Build history of the part. All positions in model axes, mm. Give positions to 0.01 mm unless a question says otherwise; leave off trailing zeros. Write each loop counter-clockwise with the first axis right and the second up, starting at its lowest first coordinate (ties: lowest second). Pieces come first, ordered by that corner, then holes.
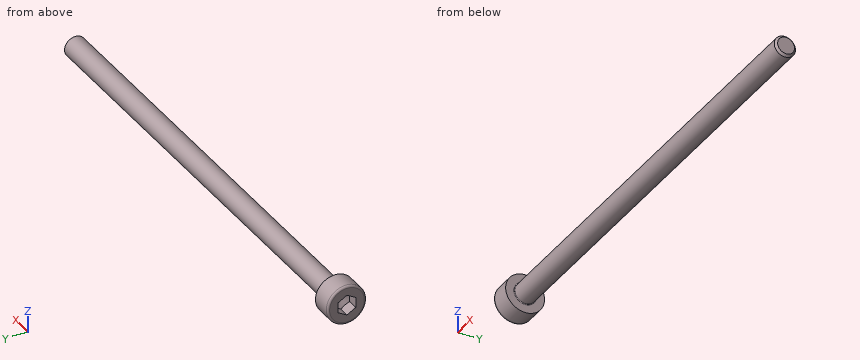
Autodesk Inventor part; units mm, degrees
ref_plane "Work Plane1" through (29, 0, 0) normal (0, -1, 0) x (1, 0, 0)
ref_plane "YZ Plane" through (0, 0, 0) normal (1, 0, 0) x (0, 1, 0)
ref_plane "XZ Plane" through (0, 0, 0) normal (0, 1, 0) x (-1, 0, 0)
sketch "Sketch1" plane through (0, 0, 0) normal (0, 0, 1) x (1, 0, 0)
  line L0 (-0.6667, 0) -> (65, 0)
  line L1 (65, 0) -> (65, 1.5)
  line L2 (65, 1.5) -> (47, 1.5)
  line L3 (47, 1.5) -> (46.6932, 1.5)
  line L4 (46.6932, 1.5) -> (0, 1.5)
  line L5 (0, 1.5) -> (0, 2.75)
  line L6 (0, 2.75) -> (-3, 2.75)
  line L7 (-3, 2.75) -> (-3, 1.4434)
  line L8 (-3, 1.4434) -> (-1.5, 1.4434)
  line L9 (-1.5, 1.4434) -> (-0.6667, 0)
  line L10 (-16.6, 0) -> (78.6, 0)
  line L11 (0, -0.55) -> (0, 3.3)
  line L12 (47, 1.5) -> (0, 1.5) construction
  dimension "d1" = 18
  dimension "d2" = 0.3068
  dimension "d3" = 3
  dimension "d4" = 1.5
  dimension "d5" = 60
  dimension "d6" = 3
  dimension "d7" = 3
  dimension "d8" = 2.8868
  dimension "d9" = 5.5
  dimension "d26" = 65
revolve "Body" add sketch "Sketch1" angle 360 about axis through (-0.6667, 0, 0) along (1, 0, 0)
sketch "Sketch2" plane through (-3, 0, 0) normal (-1, 0, 0) x (0, 0, 1)
  circle A0 centre (0, 0) radius 1.4434
  line L0 (0, -3.85) -> (0, 3.85)
  line L1 (-3.85, 0) -> (3.85, 0)
  line L2 (1.4434, 0) -> (0.7217, -1.25)
  line L3 (0.7217, -1.25) -> (-0.7217, -1.25)
  line L4 (-0.7217, -1.25) -> (-1.4434, 0)
  line L5 (-1.4434, 0) -> (-0.7217, 1.25)
  line L6 (-0.7217, 1.25) -> (0.7217, 1.25)
  line L7 (0.7217, 1.25) -> (1.4434, 0)
extrude "Slot" add sketch "Sketch2" against normal up to next contours L7 A0 | A0 L2 | L6 L0 A0 | A0 L0 L3 | L0 L6 A0 | A0 L3 L0 | L4 A0 | A0 L5
fillet "Fillet1" radius 0.3 1 edges at (-3, -2.75, 0)
thread "Thread"
chamfer "Chamfer1" distance 0.3067 distance2 0.3067 1 edges at (65, -1.5, 0) measured on face at (65, -0.92, -0.2845)
ref_plane "Work Plane1" through (29, 0, 0) normal (0, -1, 0) x (1, 0, 0)
fillet "Fillet2" radius 0.1 1 edges at (0, -1.5, 0)
equation "\"d1\" = GEL"
equation "\"d3\" = KOH"
equation "\"d4\" = INTI"
equation "\"d6\" = GD"
equation "\"d7\" = BDM"
equation "\"d8\" = 1.1547 * SW"
equation "\"d9\" = KOD"
equation "\"d26\" = NLG"
equation "\"d30\" = R"
equation "\"d17\" = RR"
equation "\"d13\" = GEL"
equation "\"d15\" = -0.5 * SPD + 0.5 * GD"
equation "\"d16\" = GUL"
equation "\"GD\" = NND"
equation "\"NLG\" = 65"
equation "\"GEL\" = 18"
equation "\"KOD\" = 5.5"
equation "\"KOH\" = 3"
equation "\"INTI\" = 1.5"
equation "\"GAL\" = 0.61345 * PTC"
equation "\"GUL\" = 0.61345 * PTC"
equation "\"BDM\" = NND"
equation "\"SW\" = 2.5"
equation "\"RR\" = 0.3"
equation "\"SPD\" = 2.38655"
equation "\"R\" = 0.1"
equation "\"TOA\" = 30deg"
equation "\"THREADDIA\" = 3"
equation "\"PTC\" = 0.5"
equation "\"NND\" = 3"
equation "\"E0\" = 1.155 * SW"
equation "\"GD1\" = THREADDIA - 1.2269 * PTC"
properties part number "ANSI B18.3.1M - M3x0.5 x 65" material "Steel, Mild"
1. Drill centre lines: line 1 along X through (y, z) = (0.35, 2); line 2 along Z through (x, y) = (40.5, 0.05). Where is each one in solid material? Low to high.
2. Drop flat-ended pins along their axis: pin 1 (2 mm diameter, centred on x = 39, y = 1.5, fed in from -Z); pin 2 (1.5 mm diameter, centred on y = 2, z = 0, fed in from +X). Give the stop position or say it passes through.
3. Saw through at A-A on x = 54.5. Give the cut face in (y, z), plus the area to 3 significant figures.
Outcome:
1. line 1: x = -3 to 0
1. line 2: z = -1.5 to 1.5
2. pin 1: stops at z = -1.41
2. pin 2: stops at x = 64.94
3. outline: circle Ø3 at (0, 0)
3. area: 7.07 mm2
